Model file for the job. Use its own axes, mm. A direction names the side the tool comes from. Give positions to 0.01 mm unless a question says otherwise; leave off trailing zeros. Order: outer loops, then holes, each group sorted by start corner. A loop starts at its lowest first (then second) coordinate and runs counter-clockwise, first axis right, second up. Notation, with made-up numbers: (-37.75, -10) -> (-17.75, -10) arc R20 cw to (-17.75, 13) -> close; hole circle Ø3 at (-16.5, 6). An arc over 180 degrees is marked (long way). Answer in a Markdown table with one row per item. Add a question column.
from build123d import *

# Parameters (mm, degrees)
SKETCH1_W           = 231.14
SKETCH1_H           = 73.66
BOSS_EXTRUDE1_DEPTH = 5.08
SKETCH2_W           = 77.046666666
SKETCH2_H           = 5.08
CUT_EXTRUDE1_DEPTH  = 6.08
SKETCH3_W           = 5.08
SKETCH3_H           = 24.553333334
CUT_EXTRUDE2_DEPTH  = 6.08
SKETCH5_W           = 2.7559
SKETCH5_H           = 13.081
CUT_EXTRUDE4_DEPTH  = 6.08
SKETCH6_W           = 6.096
SKETCH6_H           = 2.1717
CUT_EXTRUDE5_DEPTH  = 6.08


with BuildPart() as part:
    # Sketch1 → Boss-Extrude1 (new body)
    with BuildSketch(Plane.XY):
        Rectangle(SKETCH1_W, SKETCH1_H)
    extrude(amount=BOSS_EXTRUDE1_DEPTH)

    # Sketch2 → Cut-Extrude1 (cut, through all)
    with BuildSketch(Plane.XY.offset(5.08)):
        with Locations((0, -34.29)):
            Rectangle(SKETCH2_W, SKETCH2_H)
        with Locations((0, 34.29)):
            Rectangle(SKETCH2_W, SKETCH2_H)
    extrude(amount=-CUT_EXTRUDE1_DEPTH, mode=Mode.SUBTRACT)

    # Sketch3 → Cut-Extrude2 (cut, through all)
    with BuildSketch(Plane.XY.offset(5.08)):
        with Locations((-113.03, 0)):
            Rectangle(SKETCH3_W, SKETCH3_H)
        with Locations((113.03, 0)):
            Rectangle(SKETCH3_W, SKETCH3_H)
    extrude(amount=-CUT_EXTRUDE2_DEPTH, mode=Mode.SUBTRACT)

    # Sketch5 → Cut-Extrude4 (cut, through all)
    with BuildSketch(Plane.XY.offset(5.08)):
        with Locations((0, 25.2095)):
            Rectangle(SKETCH5_W, SKETCH5_H)
    extrude(amount=-CUT_EXTRUDE4_DEPTH, mode=Mode.SUBTRACT)

    # Sketch6 → Cut-Extrude5 (cut, through all)
    with BuildSketch(Plane.XY.offset(5.08)):
        with Locations((0, 25.2095)):
            Rectangle(SKETCH6_W, SKETCH6_H)
    extrude(amount=-CUT_EXTRUDE5_DEPTH, mode=Mode.SUBTRACT)


solid = part.part
Item 1: Wall check: line 1 (X direction, y = 5, z = 3.65); line 2 (Y direction, x = 14.5, z = 3.35); line 3 (X direction, y = 24, z = 1.3). Give the ranges that are in metal, low to high.
Item 2: Saw through at B-B on x = -35.5. List the corners of the cut face in (y, z).
Item 3: Two-plate mould, pull along X, no slides. Class faces 1 (the flat face through (-38.523, -34, 3)), 2 (the flat face through (-113, -12.277, 3)), 3 (the flat face through (110.49, 0, 3)), 4 (the flat face through (1.378, 21, 3)): pulls with the +X half, pulls with the -X half, needs draft (parallel to the pull), parting line crosses it, or undercut.
Item 4: Saw through at C-C on y = 7.5. List the corners of the cut face in (x, z).
Item 5: Pin check, flat tips, straight feed: pin 1 Ø0.5 at (x, z) = (2, 3) entering from -Y; pin 2 Ø2.5 at (x, z) = (-28, 1.5) entering from +Y; pin 3 Ø2 at (x, z) = (0, 1.5) entering from +Y. Stop position of each tip, or through.
Item 6: Which spindle directions (+Z, -Z, +X, -X, +Y, -Y) get a long thin tool onto all of the face, cutting with end or side? Do faces 5 (the flat face through (38.523, 34, 3)), 6 (the flat face through (-110.49, 0, 3)), 7 (the flat face through (113, -12.277, 3)). Say none if no direction does.
Evaluation:
| question | item | result |
|---|---|---|
| 1 | line 1 | x = -110.49 to 110.49 |
| 1 | line 2 | y = -31.75 to 31.75 |
| 1 | line 3 | x = -115.57 to -1.38, 1.38 to 115.57 |
| 2 | outline | (-31.75, 0) -> (31.75, 0) -> (31.75, 5.08) -> (-31.75, 5.08) -> close |
| 3 | face 1 | undercut |
| 3 | face 2 | needs draft |
| 3 | face 3 | pulls with the +X half |
| 3 | face 4 | undercut |
| 4 | outline | (-110.49, 0) -> (110.49, 0) -> (110.49, 5.08) -> (-110.49, 5.08) -> close |
| 5 | pin 1 | stops at y = -31.75 |
| 5 | pin 2 | stops at y = 31.75 |
| 5 | pin 3 | stops at y = 18.67 |
| 6 | face 5 | +Z, -Z, +Y |
| 6 | face 6 | +Z, -Z, -X |
| 6 | face 7 | +Z, -Z, +X |
